For this review, use the dimensioned drawing (mm, ordinates from the lowest corner) and the shaded views. Coordinates: 2 decimals unless noted, no trailing zeros. Loops run counter-clockwise (first coordinate to the right, second up) from the corner with the lowest first, then second, coordinate; pieces in that order, holes last.
1. To check wall thickness, follow probe 1 along Z at (x, y) = (1.65, 3.5); probe 2 along Z at (x, y) = (0.7, 5.5) (1 decimal); probe 3 along Y at (x, z) = (0.9, 4) (1 decimal). State the ranges of each line that lie inside material, in increasing order.
2. Mouldability with a two-part tool opening along Y and no side actions: class the marked faces 1, 2, 3 and 4 as pulls with the +Y half, pulls with the -Y half, needs draft (parallel to the pull), parting line crosses it, or undercut.
3. Take a section at A-A, the plane x = 1. State the section outline as (y, z) points.
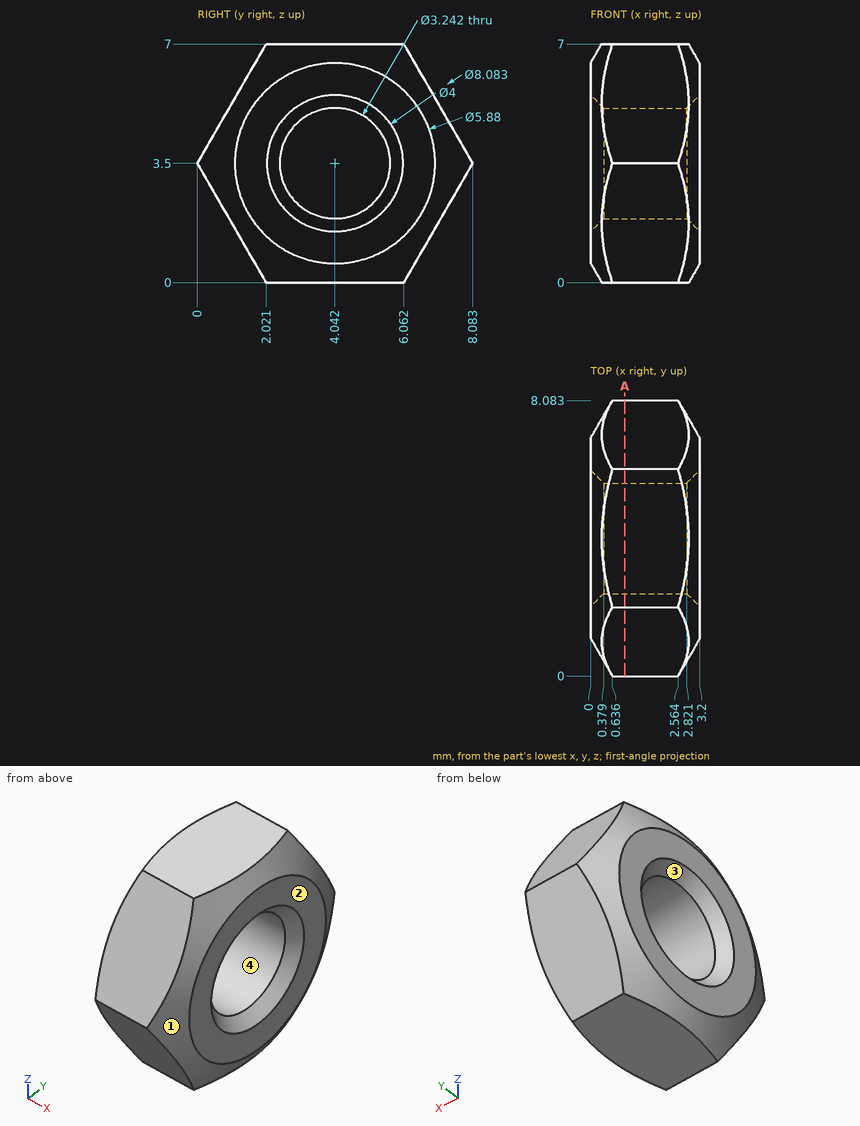
Results list:
1. probe 1: z = 0 to 1.97, 5.03 to 7
1. probe 2: z = 0 to 2.8, 4.2 to 7
1. probe 3: y = 0.3 to 2.5, 5.6 to 7.8
2. face 1: parting line crosses it
2. face 2: needs draft
2. face 3: undercut
2. face 4: undercut
3. outline: (0, 3.5) - (2.02, 0) - (6.06, 0) - (8.08, 3.5) - (6.06, 7) - (2.02, 7) - close; hole circle Ø3.24 at (4.04, 3.5)
